Can you work these out from the drawing? Everything is in mm from the part's minimum corner. Coordinates: 2 decimals unless noted, no trailing zeros. Order: outer loops, then holes, each group sorted by start corner. A loop starts at its lowest first (then second) coordinate and runs counter-clockwise, first axis right, second up. Notation, with made-up numbers: (38.25, 9) - (89.25, 9) arc R29 ccw to (89.25, 36) - close; hole circle Ø4 at (43, 37.25). An arc over 180 degrees is marked (long way). Answer as CSV lines item,"result". Start each with the question number.
Q1. I need wall thicknesses on line 1 (Z direction, x = 5, y = 1.1); line 2 (Z direction, x = 6.25, y = 4.15); line 3 (X direction, y = 2.05, z = 3.5). Which ranges of each line are inside material? Lowest first, please.
Q2. Suppose I cut it at A-A (y = 1.8). Please give me the cut outline in (x, z).
Q3. Suppose I cut it at B-B (x = 25). Please give me the cut outline in (y, z), then the cut area to 3 significant figures.
Q4. Thinking about a two-plate mould opening in Z: for the marked faces 1, 2 and 3, which applies, released by +Z, released by -Z, zero draft, split by the parting line, or undercut?
Q5. Suppose I cut it at C-C (z = 16). Please give me the cut outline in (x, y), then the cut area to 3 significant figures.
Q6. For pin 1 Ø3.5 at (x, z) = (5, 4) entering from -Y, with a flat end and sliding along its axis, tell me the tip position at first contact or that it passes through.
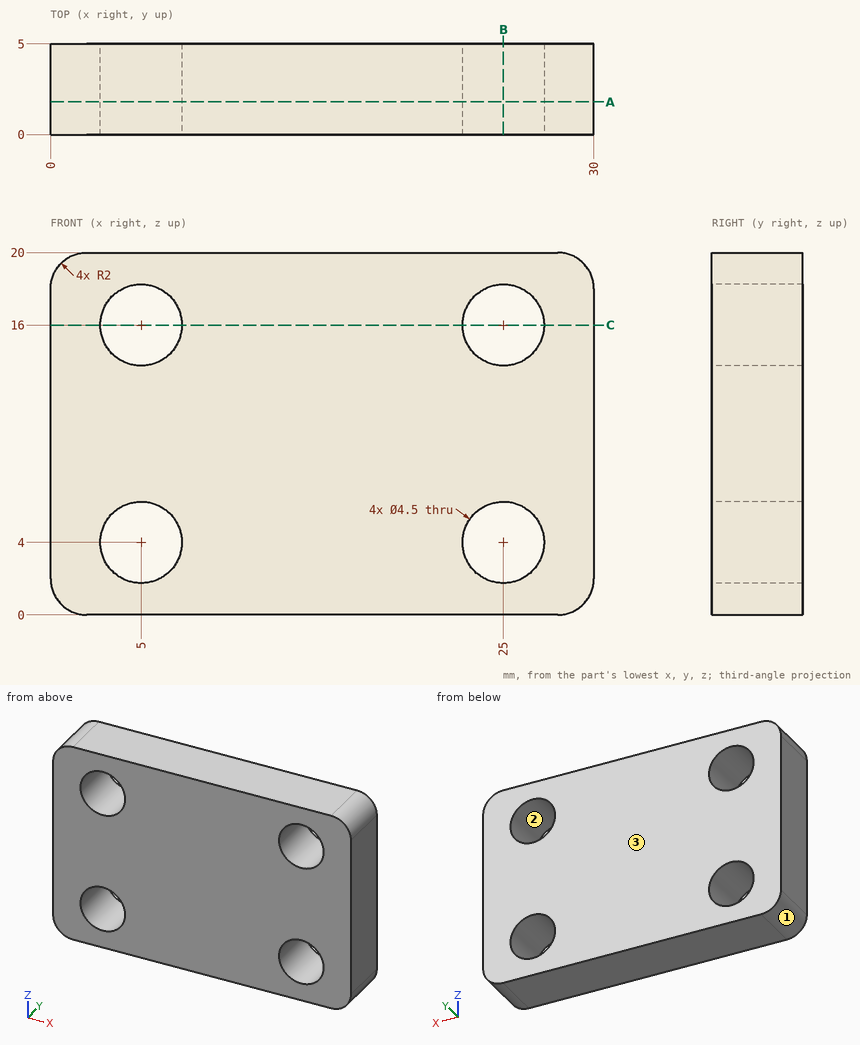
Here are the results:
1,line 1,"z = 0 to 1.75, 6.25 to 13.75, 18.25 to 20"
1,line 2,"z = 0 to 2.13, 5.87 to 14.13, 17.87 to 20"
1,line 3,"x = 0 to 2.81, 7.19 to 22.81, 27.19 to 30"
2,outline,"(0, 2) arc R2 ccw to (2, 0) - (28, 0) arc R2 ccw to (30, 2) - (30, 18) arc R2 ccw to (28, 20) - (2, 20) arc R2 ccw to (0, 18) - close; hole circle Ø4.5 at (5, 4); hole circle Ø4.5 at (5, 16); hole circle Ø4.5 at (25, 4); hole circle Ø4.5 at (25, 16)"
3,outline,"(0, 0) - (5, 0) - (5, 1.75) - (0, 1.75) - close; (0, 6.25) - (5, 6.25) - (5, 13.75) - (0, 13.75) - close; (0, 18.25) - (5, 18.25) - (5, 20) - (0, 20) - close"
3,area,"55.0 mm²"
4,face 1,"released by -Z"
4,face 2,"undercut"
4,face 3,"zero draft"
5,outline,"(0, 0) - (2.75, 0) - (2.75, 5) - (0, 5) - close; (7.25, 0) - (22.75, 0) - (22.75, 5) - (7.25, 5) - close; (27.25, 0) - (30, 0) - (30, 5) - (27.25, 5) - close"
5,area,"105 mm²"
6,pin 1,"passes through"
